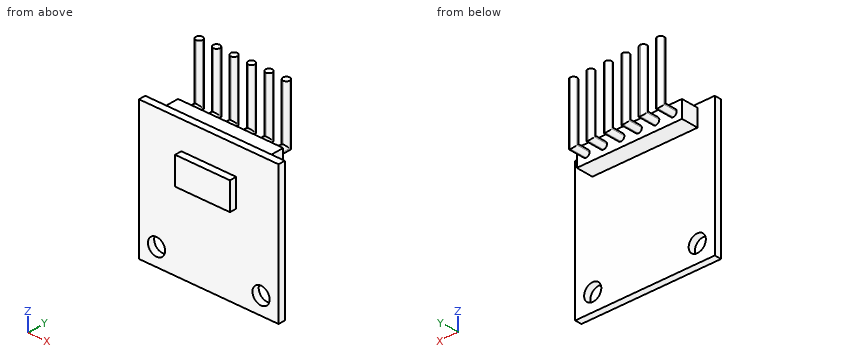
from build123d import *

# Parameters (mm, degrees)
SKETCH1_W              = 20.33
SKETCH1_H              = 20.05
SKETCH1_R              = 1.25
BOSS_EXTRUDE1_DEPTH    = 1
SKETCH2_W              = 8
SKETCH2_H              = 4
BOSS_EXTRUDE2_DEPTH    = 1
SKETCH3_W              = 15.33
SKETCH3_H              = 2.5
BOSS_EXTRUDE3_DEPTH    = 2.5
SKETCH4_W              = 1
SKETCH4_H              = 1
BOSS_EXTRUDE4_DEPTH    = 2.5
SKETCH5_W              = 1
SKETCH5_H              = 1
BOSS_EXTRUDE5_DEPTH    = 8
FILLET1_R              = 0.5
LPATTERN4_COUNT        = 6
LPATTERN4_PITCH        = 2.54
FILLET1_OF_LPATTERN4_R = 0.5


with BuildPart() as part:
    # Sketch1 → Boss-Extrude1 (new body)
    with BuildSketch(Plane(origin=(0, 0, 0), x_dir=(1, 0, 0), z_dir=(0, 1, 0))):
        Rectangle(SKETCH1_W, SKETCH1_H)
        with Locations(Location((-7.615, 7.475, 0), (0, 0, 270))):
            Circle(SKETCH1_R, mode=Mode.SUBTRACT)
        with Locations(Location((7.615, 7.475, 0), (0, 0, 90))):
            Circle(SKETCH1_R, mode=Mode.SUBTRACT)
    extrude(amount=BOSS_EXTRUDE1_DEPTH)

    # Sketch2 → Boss-Extrude2 (add)
    with BuildSketch(Plane.XZ):
        with Locations((0, 3.975)):
            Rectangle(SKETCH2_W, SKETCH2_H)
    extrude(amount=BOSS_EXTRUDE2_DEPTH)

    # Sketch3 → Boss-Extrude3 (add)
    with BuildSketch(Plane(origin=(0, 1, 0), x_dir=(1, 0, 0), z_dir=(0, 1, 0))):
        with Locations((0, -8.275)):
            Rectangle(SKETCH3_W, SKETCH3_H)
    extrude(amount=BOSS_EXTRUDE3_DEPTH)

    # Sketch4 → Boss-Extrude4 (add)
    with BuildSketch(Plane(origin=(0, 3.5, 0), x_dir=(1, 0, 0), z_dir=(0, 1, 0))):
        with Locations((-6.395, -8.255)):
            Rectangle(SKETCH4_W, SKETCH4_H)
    boss_extrude4 = extrude(amount=BOSS_EXTRUDE4_DEPTH)

    # Sketch5 → Boss-Extrude5 (add)
    with BuildSketch(Plane.XY.offset(8.755)):
        with Locations((-6.395, 5.5)):
            Rectangle(SKETCH5_W, SKETCH5_H)
    boss_extrude5 = extrude(amount=BOSS_EXTRUDE5_DEPTH)

    # Fillet1
    fillet1_edges = [part.edges().sort_by_distance(p)[0] for p in [
        (-5.895, 5, 12.755),
        (-6.895, 5, 12.755),
        (-5.895, 4.25, 8.755),
        (-6.895, 4.25, 8.755),
        (-5.895, 4.75, 7.755),
        (-6.895, 4.75, 7.755),
        (-5.895, 6, 12.255),
        (-6.895, 6, 12.255),
    ]]
    fillet(fillet1_edges, radius=FILLET1_R - 0.0001)  # a hair under: the kernel refuses the full size

    # LPattern4: Boss-Extrude4, Boss-Extrude5 ×6
    with Locations(*[(i * LPATTERN4_PITCH, 0, 0) for i in range(1, LPATTERN4_COUNT)]):
        add(boss_extrude4)
        add(boss_extrude5)

    # Fillet1 of LPattern4
    fillet1_of_lpattern4_edges = [part.edges().sort_by_distance(p)[0] for p in [
        (-3.355, 5, 12.755),
        (-4.355, 5, 12.755),
        (-3.355, 4.25, 8.755),
        (-4.355, 4.25, 8.755),
        (-3.355, 4.75, 7.755),
        (-4.355, 4.75, 7.755),
        (-3.355, 6, 12.255),
        (-4.355, 6, 12.255),
        (-0.815, 5, 12.755),
        (-1.815, 5, 12.755),
        (-0.815, 4.25, 8.755),
        (-1.815, 4.25, 8.755),
        (-0.815, 4.75, 7.755),
        (-1.815, 4.75, 7.755),
        (-0.815, 6, 12.255),
        (-1.815, 6, 12.255),
        (1.725, 5, 12.755),
        (0.725, 5, 12.755),
        (1.725, 4.25, 8.755),
        (0.725, 4.25, 8.755),
        (1.725, 4.75, 7.755),
        (0.725, 4.75, 7.755),
        (1.725, 6, 12.255),
        (0.725, 6, 12.255),
        (4.265, 5, 12.755),
        (3.265, 5, 12.755),
        (4.265, 4.25, 8.755),
        (3.265, 4.25, 8.755),
        (4.265, 4.75, 7.755),
        (3.265, 4.75, 7.755),
        (4.265, 6, 12.255),
        (3.265, 6, 12.255),
        (6.805, 5, 12.755),
        (5.805, 5, 12.755),
        (6.805, 4.25, 8.755),
        (5.805, 4.25, 8.755),
        (6.805, 4.75, 7.755),
        (5.805, 4.75, 7.755),
        (6.805, 6, 12.255),
        (5.805, 6, 12.255),
    ]]
    fillet(fillet1_of_lpattern4_edges, radius=FILLET1_OF_LPATTERN4_R - 0.0001)  # a hair under: the kernel refuses the full size


solid = part.part
Can you work these out from the model? Positions are in its coordinate system, mm. Coordinates: 2 decimals unless noted, no trailing zeros. Loops run counter-clockwise (first coordinate to the right, second up) from the corner with the lowest first, then second, coordinate; pieces in that order, holes last. Notation, with made-up numbers: M -17.5,44.25 L 1.5,44.25 A36 cw 1.5,81.25 Z; hole C -22.75,58 d1. An arc over 180 degrees is marked long. Return JSON: item names as keys, results as strings. Group by question number.
Item 1: Imagine slicing it at C-C (z = -7.5). Please give me the cut outline in (x, y) (3 decimals), and give its area (3 significant figures).
Item 2: Imagine slicing it at A-A (x = -5.25). Please give me the cut outline in (y, z) (3 decimals).
Item 3: I'm going to push flat-ended pins straight in: pin 1 Ø1.5 at (x, y) = (-1.5, 5) entering from +Z (3 decimals); pin 2 Ø2 at (y, z) = (4.5, 11) entering from +X (3 decimals); pin 3 Ø1.2 at (y, z) = (2.5, 8.5) entering from -X (3 decimals); pin 4 Ø6 at (x, z) = (-2, -1.5) entering from +Y. Where does each tip first touch, or does it pass through?
Item 4: Imagine slicing it at B-B (z = 11). Give the number of separate pieces and of enclosed holes in the cut face, and give its area (3 significant figures).
Item 5: Imagine slicing it at D-D (y = 2.75). Please give me the cut outline in (x, z) (3 decimals), and give its area (3 significant figures).
Item 6: If I drill on L1, parallel to Y at x = 4.25, z = -4; L2, parallel to Z at x = 1.5, y = 2 (3 decimals); L3, parallel to Y at x = -3, z = 8, over which ranges is the centre line in solid material (lowest first)? Write a range as from..to.
Verdict:
{
 "1": {"outline": "M -10.165,0 L -8.865,0 L -8.865,1 L -10.165,1 Z; M -6.365,0 L 6.365,0 L 6.365,1 L -6.365,1 Z; M 8.865,0 L 10.165,0 L 10.165,1 L 8.865,1 Z", "area": "15.3 mm^2"},
 "2": {"outline": "M 0,-10.025 L 1,-10.025 L 1,7.025 L 3.5,7.025 L 3.5,9.525 L 1,9.525 L 1,10.025 L 0,10.025 Z"},
 "3": {"pin 1": "stops at z = 16.755", "pin 2": "stops at x = 6.805", "pin 3": "stops at x = -7.665", "pin 4": "stops at y = 1"},
 "4": {"separate pieces": "6", "enclosed holes": "0", "area": "4.71 mm^2"},
 "5": {"outline": "M -7.665,7.025 L 7.665,7.025 L 7.665,9.525 L -7.665,9.525 Z", "area": "38.3 mm^2"},
 "6": {"L1": "y = 0..1", "L2": "z = 7.025..9.525", "L3": "y = 0..3.5"}
}
